from build123d import *

# Parameters (mm, degrees)
EXTRUDE_THIN2_DEPTH            = 9.0043
SKETCH4_R                      = 2.2479
CUT_EXTRUDE2_DEPTH             = 86.321916719
CHAMFER1_SIZE                  = 2.2479
CHAMFER1_SIZE_2                = 2.024018251
CIRPATTERN2_COUNT              = 2
CIRPATTERN2_ANGLE              = 180
CHAMFER1_OF_CIRPATTERN2_SIZE   = 2.024018251
CHAMFER1_OF_CIRPATTERN2_SIZE_2 = 2.2479


with BuildPart() as part:
    # Sketch3 → Extrude-Thin2 (new, symmetric)
    with BuildSketch(Plane(origin=(0, 0, 0), x_dir=(1, 0, 0), z_dir=(0, 1, 0))):
        with BuildLine():
            Line((0, -59.9948), (0, -2.4003))
            ThreePointArc((0, -2.4003), (0.703031593, -0.703031593), (2.4003, 0))
            Line((2.4003, 0), (59.9948, 0))
            Line((59.9948, 0), (59.9948, -1.6002))
            Line((59.9948, -1.6002), (2.4003, -1.6002))
            ThreePointArc((2.4003, -1.6002), (1.834543864, -1.834543864), (1.6002, -2.4003))
            Line((1.6002, -2.4003), (1.6002, -59.9948))
            Line((1.6002, -59.9948), (0, -59.9948))
        make_face()
    extrude(amount=EXTRUDE_THIN2_DEPTH, both=True)

    # Sketch4 → Cut-Extrude2 (cut, through all)
    with BuildSketch(Plane.XY):
        with Locations(Location((46.7975, 1.5875, 0), (0, 0, 180))):
            Circle(SKETCH4_R)
        with Locations(Location((14.7975, -1.5875, 0), (0, 0, 180))):
            Circle(SKETCH4_R)
    cut_extrude2 = extrude(amount=CUT_EXTRUDE2_DEPTH, mode=Mode.SUBTRACT)

    # Chamfer1
    # the kernel refuses this chamfer: 2.2479, 2.024018251 mm, written as the material it takes off along each edge
    with BuildSketch(Plane(origin=(46.7975, 1.5875, 1.6002), x_dir=(-1, 0, 0), z_dir=(0, -1, 0))) as chamfer1_piece_1:
        Polygon((2.2479 + CHAMFER1_SIZE, 0), (2.2479, CHAMFER1_SIZE_2), (2.2479, 0), align=None)
    revolve(axis=Axis((46.7975, 1.5875, 1.6002), (0, 0, -1)), mode=Mode.SUBTRACT)
    with BuildSketch(Plane(origin=(14.7975, -1.5875, 1.6002), x_dir=(-1, 0, 0), z_dir=(0, -1, 0))) as chamfer1_piece_2:
        Polygon((2.2479 + CHAMFER1_SIZE, 0), (2.2479, CHAMFER1_SIZE_2), (2.2479, 0), align=None)
    revolve(axis=Axis((14.7975, -1.5875, 1.6002), (0, 0, -1)), mode=Mode.SUBTRACT)

    # CirPattern2: Cut-Extrude2 ×2 about axis
    cirpattern2_axis = Axis((0, 0, 0), (0.7071067811865462, 0, 0.7071067811865489))
    for i in range(1, CIRPATTERN2_COUNT):
        add(cut_extrude2.rotate(cirpattern2_axis, i * CIRPATTERN2_ANGLE / (CIRPATTERN2_COUNT - 1)), mode=Mode.SUBTRACT)

    # Chamfer1 of CirPattern2
    # the kernel refuses this chamfer: 2.2479, 2.024018251 mm, written as the material it takes off along each edge
    with BuildSketch(Plane(origin=(1.6002, -1.5875, 46.7975), x_dir=(0, 0, -1), z_dir=(0, 1, 0))) as chamfer1_of_cirpattern2_piece_1:
        Polygon((2.2479, CHAMFER1_OF_CIRPATTERN2_SIZE), (2.2479 + CHAMFER1_OF_CIRPATTERN2_SIZE_2, 0), (2.2479, 0), align=None)
    revolve(axis=Axis((1.6002, -1.5875, 46.7975), (-1, 0, 0)), mode=Mode.SUBTRACT)
    with BuildSketch(Plane(origin=(1.6002, 1.5875, 14.7975), x_dir=(0, 0, -1), z_dir=(0, 1, 0))) as chamfer1_of_cirpattern2_piece_2:
        Polygon((2.2479, CHAMFER1_OF_CIRPATTERN2_SIZE), (2.2479 + CHAMFER1_OF_CIRPATTERN2_SIZE_2, 0), (2.2479, 0), align=None)
    revolve(axis=Axis((1.6002, 1.5875, 14.7975), (-1, 0, 0)), mode=Mode.SUBTRACT)


solid = part.part
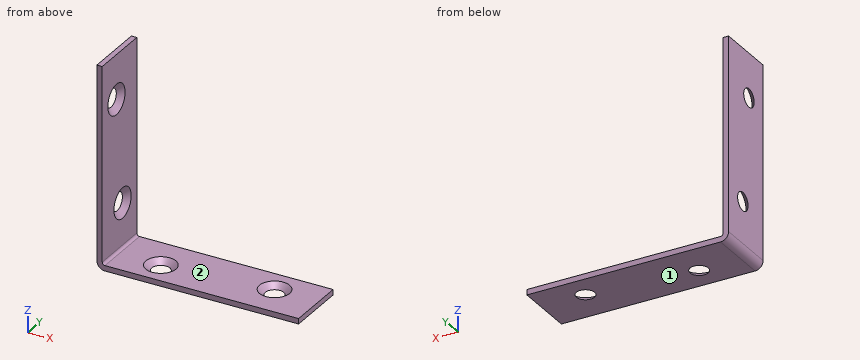
Source: CAD feature listing. Evaluate the final solid. Frame: model axes, mm. Face numbers are marked on the shaded views. A direction names the side the tool comes from. Round coordinates to 2 decimals unless told otherwise and drop trailing zeros. Write each loop counter-clockwise with the first axis right and the second up, starting at its lowest first coordinate (ties: lowest second). Pieces come first, ordered by that corner, then holes. Notation, with made-up numbers: M 40,44.5 L 70,44.5 A22 cw 70,83.5 Z; hole C 64,21 d4. An arc over 180 degrees is marked long. One line per item, written item: value. Start each with the question number.
Item 1: Section query B-B (x = 29.5). Return the cut outline in (y, z), plus the area to 3 significant figures.
Item 2: Section query A-A (y = -7.5). Return the cut outline in (x, z), plus the area to 3 significant figures.
Item 3: Pin query (flat end, axial travel): pin 1 (5 mm diameter, centred on x = 31, y = 5, fed in from +Z). Return the tip coordinate at first contact, or that it passes through.
Item 4: Ray query, L1, parallel to Z at x = 46, y = -8; L2, parallel to Z at x = 46.5, y = -2.25. Return the intervals inside material, ascending. Write a range as from..to.
Item 5: Section query D-D (y = 0.25). State how many separate pieces and enclosed holes the cut face has, plus the area to 3 significant figures.
Item 6: Section query C-C (z = 39.5). Return the cut outline in (x, y).
Item 7: Set-up query: the marked faces 1 and 2. Return all of +Z, -Z, +X, -X, +Y, -Y with unobstructed straight access to the full face (end or side cutting, diameter ignored); none if empty.
Result set:
1. outline: M -9,0 L 9,0 L 9,1.6 L -9,1.6 Z
1. area: 28.8 mm²
2. outline: M 0,2.4 A2.4 ccw 2.4,0 L 59.99,0 L 59.99,1.6 L 2.4,1.6 A0.8 cw 1.6,2.4 L 1.6,59.99 L 0,59.99 Z
2. area: 188 mm²
3. pin 1: stops at z = 1.6
4. L1: z = 0..1.6
4. L2: z = 0..1.02
5. separate pieces: 5
5. enclosed holes: 0
5. area: 147 mm²
6. outline: M 0,-9 L 1.6,-9 L 1.6,9 L 0,9 Z
7. face 1: -Z, +X, -X, +Y, -Y
7. face 2: +Z, +X, +Y, -Y
